Input: part model. Units: mm. Frame: model coordinates. Face numbers are marked on the shaded views. Coordinates: 2 decimals unless noted, no trailing zeros. Order: outer loops, then holes, each group sorted by start corner. A loop starts at its lowest first (then second) coordinate and runs counter-clockwise, first axis right, second up. Notation, with made-up numbers: (17.25, 49.25) -> (70.25, 49.25) arc R18 ccw to (70.25, 84.25) -> close; hole circle Ø8 at (67, -34.75). An arc over 180 degrees is marked (long way). One line per item, written item: value. Start each with the question number.
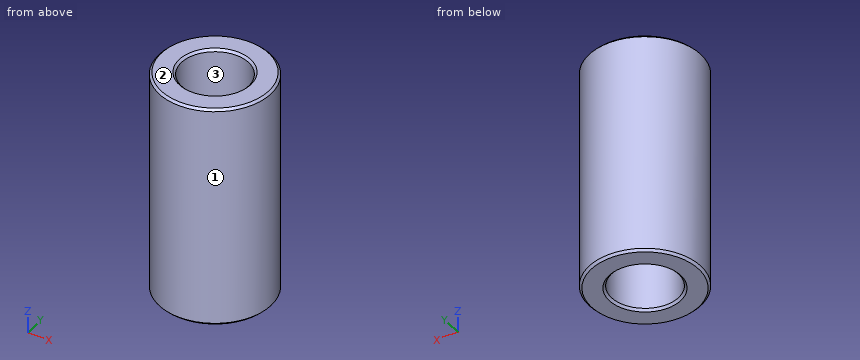
Autodesk Inventor part; units mm, degrees
ref_plane "YZ Plane" through (0, 0, 0) normal (1, 0, 0) x (0, 1, 0)
ref_plane "XZ Plane" through (0, 0, 0) normal (0, 1, 0) x (-1, 0, 0)
ref_plane "XY Plane" through (0, 0, 0) normal (0, 0, 1) x (1, 0, 0)
sketch "Sketch1" plane through (0, 0, 0) normal (0, 0, 1) x (1, 0, 0)
  circle A0 centre (0, 0) radius 2.5
  circle A1 centre (0, 0) radius 1.5
  dimension "d0" = 5
  dimension "d1" = 3
extrude "Extrusion1" add sketch "Sketch1" along normal mid plane 10
thread "Thread1"
thread "Thread2"
chamfer "Chamfer1" distance 0.1 angle 45 4 edges at (-2.5, 0, 5) (-1.5, 0, 5) (-1.5, 0, -5) (-2.5, 0, -5)
properties part number "M3 10mm Standoff" material "Aluminum 6061"
1) Mould query, pull axis X, two halves, no side actions, for the marked faces 1, 2 and 3. Classes: +X half, -X half, draft (parallel to the pull), parting line (faces both ways), or undercut.
2) Pin query (flat end, axial travel): pin 1 Ø1 at (y, z) = (-2, -3) entering from +X. Return the tip coordinate at first contact, or that it passes through.
3) Ray query, line 1 along Y through (x, z) = (0, 1.25); line 2 along Y through (x, z) = (-0.6, 1.25). Return the intervals inside material, ascending. Write a range as from..to.
4) Section query C-C, the plane z = 3. Return the cut outline in (x, y), plus the area to 3 significant figures.
5) Section query A-A, the plane x = 0. Return the cut outline in (y, z), plus the area to 3 significant figures.
Entries:
1. face 1: parting line
1. face 2: draft
1. face 3: undercut
2. pin 1: stops at x = 2
3. line 1: y = -2.5..-1.5, 1.5..2.5
3. line 2: y = -2.43..-1.37, 1.37..2.43
4. outline: circle Ø5 at (0, 0); hole circle Ø3 at (0, 0)
4. area: 12.6 mm2
5. outline: (-2.5, -4.9) -> (-2.4, -5) -> (-1.6, -5) -> (-1.5, -4.9) -> (-1.5, 4.9) -> (-1.6, 5) -> (-2.4, 5) -> (-2.5, 4.9) -> close; (1.5, -4.9) -> (1.6, -5) -> (2.4, -5) -> (2.5, -4.9) -> (2.5, 4.9) -> (2.4, 5) -> (1.6, 5) -> (1.5, 4.9) -> close
5. area: 20.0 mm2
